```python
from build123d import *

# Parameters (mm, degrees)
BOSS_EXTRUDE1_DEPTH = 1
FILLET2_R           = 3
FILLET3_R           = 12
SKETCH2_R           = 2
CUT_EXTRUDE1_DEPTH  = 1
SKETCH3_R           = 14.5
BOSS_EXTRUDE2_DEPTH = 8
BOSS_EXTRUDE2_TAPER = 14
SKETCH6_R           = 12.505375977
BOSS_EXTRUDE4_DEPTH = 3.5
BOSS_EXTRUDE4_TAPER = 38
SKETCH7_R           = 9.770876284
BOSS_EXTRUDE5_DEPTH = 1
BOSS_EXTRUDE5_TAPER = 66


# Read off the part's stored shape, not the designer's step: Dome4
with BuildPart() as part:
    # Sketch1 → Boss-Extrude1 (new body)
    with BuildSketch(Plane(origin=(0, 0, 0), x_dir=(1, 0, 0), z_dir=(0, 1, 0))):
        Polygon((-26.05, -2.94e-07), (0, 19.1), (26.05, 2.94e-07), (0, -19.1), align=None)
    extrude(amount=BOSS_EXTRUDE1_DEPTH)

    # Fillet2
    fillet2_edges = [part.edges().sort_by_distance(p)[0] for p in [
        (26.05, 0.5, -2.94e-07),
        (-26.05, 0.5, 2.94e-07),
    ]]
    fillet(fillet2_edges, radius=FILLET2_R)

    # Fillet3
    fillet3_edges = [part.edges().sort_by_distance(p)[0] for p in [
        (0, 0.5, 19.1),
        (0, 0.5, -19.1),
    ]]
    fillet(fillet3_edges, radius=FILLET3_R)

    # Sketch2 → Cut-Extrude1 (cut)
    with BuildSketch(Plane(origin=(0, 1, 0), x_dir=(1, 0, 0), z_dir=(0, 1, 0))):
        with Locations(Location((-19.996075031, 0.396211257, 0), (0, 0, 270))):
            Circle(SKETCH2_R)
        with Locations(Location((19.996075025, 0.39621155, 0), (0, 0, 270))):
            Circle(SKETCH2_R)
    extrude(amount=-CUT_EXTRUDE1_DEPTH, mode=Mode.SUBTRACT)

    # Sketch3 → Boss-Extrude2 (add)
    with BuildSketch(Plane(origin=(0, 1, 0), x_dir=(1, 0, 0), z_dir=(0, 1, 0))):
        Circle(SKETCH3_R)
    extrude(amount=BOSS_EXTRUDE2_DEPTH, taper=BOSS_EXTRUDE2_TAPER)

    # Sketch6 → Boss-Extrude4 (add)
    with BuildSketch(Plane(origin=(0, 9, 0), x_dir=(1, 0, 0), z_dir=(0, 1, 0))):
        Circle(SKETCH6_R)
    extrude(amount=BOSS_EXTRUDE4_DEPTH, taper=BOSS_EXTRUDE4_TAPER)

    # Sketch7 → Boss-Extrude5 (add)
    with BuildSketch(Plane(origin=(0, 12.5, 0), x_dir=(1, 0, 0), z_dir=(0, 1, 0))):
        Circle(SKETCH7_R)
    extrude(amount=BOSS_EXTRUDE5_DEPTH, taper=BOSS_EXTRUDE5_TAPER)

    # Dome4 outline → Dome4 (revolve)
    with BuildSketch(Plane.XY):
        with BuildLine():
            Line((0, 13.5), (7.524839511, 13.499999992))
            ThreePointArc((7.524839511, 13.499999992), (5.312090214, 18.804802861), (0, 21))
            Line((0, 21), (0, 13.5))
        make_face()
    revolve(axis=Axis((0, 0, 0), (0, 1, 0)))


solid = part.part
```
CAD build for the part. Positions are in the model's coordinates, mm. A direction names the side the tool comes from. Round coordinates to 2 decimals unless told otherwise and drop trailing zeros. Order: outer loops, then holes, each group sorted by start corner. A loop starts at its lowest first (then second) coordinate and runs counter-clockwise, first axis right, second up. Notation, with made-up numbers: (13.5, -11) -> (18.5, -11) arc R22 cw to (18.5, 11) -> close; hole circle Ø4 at (18, 66.25). An arc over 180 degrees is marked (long way). One line per question, with ' | ' between items.
Q1. Probe probe 1 along Y at (x, z) = (22, 1.5); probe 2 along Z at (x, y) = (-6, 16.25); probe 3 along X at (y, z) = (4.5, -7). List the from-to ranges inside material, lowest first.
Completed:
probe 1: y = 0 to 1 | probe 2: z = -3.59 to 3.59 | probe 3: x = -11.69 to 11.69
Q2. Slice it at B-B (z = 0). Give the number of separate pieces and of enclosed holes in the cut face, then the cut area to 3 significant figures.
Completed:
separate pieces: 3 | enclosed holes: 0 | area: 440 mm^2
Q3. Slice it at C-C (y = 18.75). Write the cut outline in (x, z), then the cut area to 3 significant figures.
Completed:
outline: circle Ø10.73 at (0, 0) | area: 90.5 mm^2
Q4. Two-plate mould, pull along X, no slides. Class faces 3 (the flat face through (14.81, 0.49, -8.24)), 4 (the cylindrical face through (-23.976, 0.507, -0.039)), 5 (the cylindrical face through (18.044, 0.507, -0.83)), 6 (the cylindrical face through (-18.013, 0.507, -0.657)): released by +X, released by -X, zero draft, split by the parting line, or undercut.
Completed:
face 3: released by +X | face 4: released by -X | face 5: undercut | face 6: undercut
Q5. Slice it at D-D (x = -17). Write the cut outline in (y, z), then the cut area to 3 significant figures.
Completed:
outline: (0, -6.64) -> (1, -6.64) -> (1, 6.64) -> (0, 6.64) -> close | area: 13.3 mm^2
Q6. Slice it at A-A (x = 0). Write the cut outline in (y, z).
Completed:
outline: (0, -16.22) -> (1, -16.22) -> (1, -14.5) -> (9, -12.51) -> (12.5, -9.77) -> (13.5, -7.52) arc R7.52 ccw to (13.5, 7.52) -> (12.5, 9.77) -> (9, 12.51) -> (1, 14.5) -> (1, 16.22) -> (0, 16.22) -> close
Q7. Drop flat-ended pins along their axis: pin 1 (5 mm diameter, centred on x = -12.5, y = 7.5, fed in from +Z); pin 2 (1 mm diameter, centred on y = 17, z = 2, fed in from +X); pin 3 (9.5 mm diameter, centred on x = -4.5, z = 4, fed in from +Y). Give the stop position or say it passes through.
Completed:
pin 1: stops at z = 8.27 | pin 2: stops at x = 6.63 | pin 3: stops at y = 20.89
Q8. Which spindle directions (+Z, -Z, +X, -X, +Y, -Y) get a long thin tool onto all of the face, cutting with end or side? Do faces 1 (the flat face through (13, 1, -7)), 2 (the cylindrical face through (23.976, 0.507, -0.039)). Say none if no direction does.
Completed:
face 1: +Y | face 2: +X, +Y, -Y
